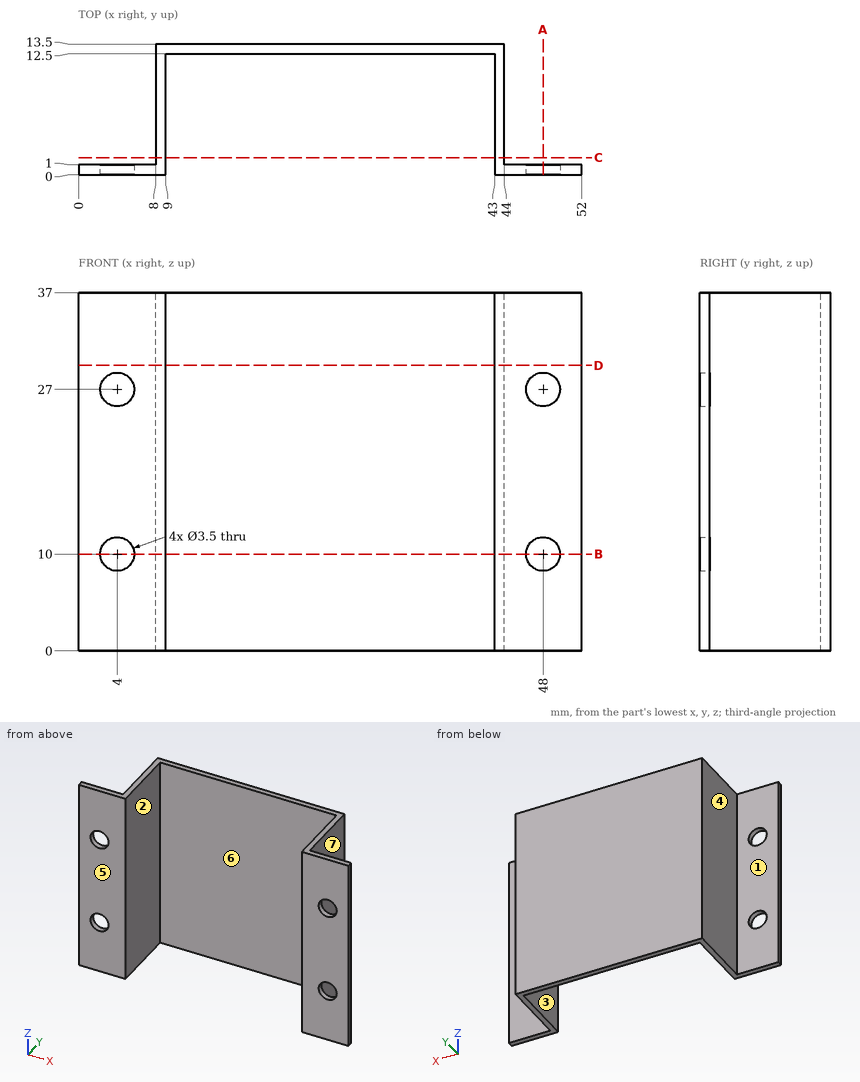
Check sheet for the drawn part. Datum: minimum x, y, z corner. Units: mm. A direction names the side the tool comes from. Coordinates: 2 decimals unless noted, no trailing zeros. Loops run counter-clockwise (first coordinate to the right, second up) from the corner with the lowest first, then second, coordinate; pieces in that order, holes last. Notation, with made-up numbers: (79, 35) -> (92, 35) arc R25 ccw to (92, 53) -> close; hole circle Ø1 at (6.5, 61.5). An arc over 180 degrees is marked (long way). Answer as a JSON object with one key per item and string values. Group by question number.
Item 1: Tool access check on the marked faces 5, 6 and 7. Record the directions out of +Z, -Z, +X, -X, +Y, -Y that give a thin tool (end or side, any length) a straight path to the whole face; none if there is none.
Item 2: Sectioned sample at A-A on x = 48. Record the boundary of the cut face in (y, z).
Item 3: Sectioned sample at C-C on y = 1.75. Record the boundary of the cut face in (x, z), plus the area to 3 significant figures.
Item 4: Mould release check, pull along X, two halves, no side actions. Record for the marked faces 1, 2, 3 and 4: +X half, -X half, draft (parallel to the pull), parting line (faces both ways), or undercut.
Item 5: Sectioned sample at B-B on z = 10. Record the boundary of the cut face in (x, y).
Item 6: Scan lines: probe 1 along X at (y, z) = (0.75, 10); probe 2 along Z at (x, y) = (48, 0.4); probe 3 along X at (y, z) = (11.5, 35). Record each from-to range of solid material in increasing order.
Item 7: Depth check by flat-ended pin: pin 1 (3 mm diameter, centred on x = 4, z = 27, fed in from -Y); pin 2 (5.5 mm diameter, centred on x = 4, z = 10, fed in from -Y); pin 3 (5 mm diameter, centred on y = 9, z = 7.5, fed in from +X); pin 4 (4 mm diameter, centred on x = 19, z = 18.5, fed in from -Y). Enter the tip coordinate at first touch or a pass-through.
Item 8: Sectioned sample at D-D on z = 29.5. Record the boundary of the cut face in (x, y).
Evaluation:
{
 "1": {"face 5": "+Z, -Z, +X, -X, -Y", "face 6": "+Z, -Z, -Y", "face 7": "+Z, -Z, +X, +Y"},
 "2": {"outline": "(0, 0) -> (1, 0) -> (1, 8.25) -> (0, 8.25) -> close; (0, 11.75) -> (1, 11.75) -> (1, 25.25) -> (0, 25.25) -> close; (0, 28.75) -> (1, 28.75) -> (1, 37) -> (0, 37) -> close"},
 "3": {"outline": "(8, 0) -> (9, 0) -> (9, 37) -> (8, 37) -> close; (43, 0) -> (44, 0) -> (44, 37) -> (43, 37) -> close", "area": "74.0 mm²"},
 "4": {"face 1": "draft", "face 2": "undercut", "face 3": "undercut", "face 4": "-X half"},
 "5": {"outline": "(0, 0) -> (2.25, 0) -> (2.25, 1) -> (0, 1) -> close; (5.75, 0) -> (9, 0) -> (9, 12.5) -> (43, 12.5) -> (43, 0) -> (46.25, 0) -> (46.25, 1) -> (44, 1) -> (44, 13.5) -> (8, 13.5) -> (8, 1) -> (5.75, 1) -> close; (49.75, 0) -> (52, 0) -> (52, 1) -> (49.75, 1) -> close"},
 "6": {"probe 1": "x = 0 to 2.25, 5.75 to 9, 43 to 46.25, 49.75 to 52", "probe 2": "z = 0 to 8.25, 11.75 to 25.25, 28.75 to 37", "probe 3": "x = 8 to 9, 43 to 44"},
 "7": {"pin 1": "passes through", "pin 2": "stops at y = 0", "pin 3": "stops at x = 44", "pin 4": "stops at y = 12.5"},
 "8": {"outline": "(0, 0) -> (9, 0) -> (9, 12.5) -> (43, 12.5) -> (43, 0) -> (52, 0) -> (52, 1) -> (44, 1) -> (44, 13.5) -> (8, 13.5) -> (8, 1) -> (0, 1) -> close"}
}
